from build123d import *

# Parameters (mm, degrees)
F1_DEPTH = 63.5
F2_DEPTH = 25.4
F3_DEPTH = 10.4775
F0_W     = 25.4
F0_H     = 4.7752
F0_H_2   = 19.05
F0_H_3   = 4.7498
F5_R     = 5.08


with BuildPart() as f1:
    # F0 (on Front) → F1 (new body, symmetric)
    with BuildSketch(Plane.XZ):
        Polygon((22.225, 9.525), (-41.275, 9.525), (-41.275, -9.525), (41.275, -9.525), (41.275, 9.525), align=None)
    extrude(amount=F1_DEPTH, both=True)

    # F0 (on Front) → F2 (join, symmetric)
    with BuildSketch(Plane.XZ):
        Polygon((22.225, 9.525), (-41.275, 9.525), (-41.275, -9.525), (41.275, -9.525), (41.275, 9.525), align=None)
        with BuildLine():
            Line((22.225, 27.0002), (22.225, 9.525))
            Line((22.225, 9.525), (41.275, 9.525))
            Line((41.275, 9.525), (41.275, 27.0002))
            ThreePointArc((41.275, 27.0002), (45.9246798487, 38.2255201513), (57.15, 42.8752))
            Line((57.15, 42.8752), (85.725, 42.8752))
            Line((85.725, 42.8752), (85.725, 61.9252))
            Line((85.725, 61.9252), (57.15, 61.9252))
            ThreePointArc((57.15, 61.9252), (32.4542956671, 51.6959043329), (22.225, 27.0002))
        make_face()
    extrude(amount=F2_DEPTH, both=True)

    # F0 (on Front) → F3 (join, symmetric)
    with BuildSketch(Plane.XZ):
        with BuildLine():
            add(Edge.make_bspline(
                [(-41.275, 9.525), (-41.4362549782, 59.2387728393), (7.6155788265, 61.9246140122), (57.15, 61.9252)],
                knots=[0, 0, 0, 0, 111.5045361635, 111.5045361635, 111.5045361635, 111.5045361635], degree=3))
            Line((-41.275, 9.525), (22.225, 9.525))
            Line((22.225, 9.525), (22.225, 27.0002))
            ThreePointArc((22.225, 27.0002), (32.4542956671, 51.6959043329), (57.15, 61.9252))
        make_face()
    extrude(amount=F3_DEPTH, both=True)

    # F0 (on Front) → F4 (revolve)
    with BuildSketch(Plane.XZ):
        with Locations((98.425, 40.4876)):
            Rectangle(F0_W, F0_H)
        with Locations((98.425, 52.4002)):
            Rectangle(F0_W, F0_H_2)
        with Locations((98.425, 64.3001)):
            Rectangle(F0_W, F0_H_3)
    revolve(axis=Axis((85.725, 0, 52.3875), (0, 0, 1)))

    # F5
    f5_edges = [f1.edges().sort_by_distance(p)[0] for p in [
        (41.275, 63.5, 0),
        (-41.275, 63.5, 0),
        (-41.275, -63.5, 0),
        (41.275, -63.5, 0),
    ]]
    fillet(f5_edges, radius=F5_R)


solid = f1.part
Model file for the job. Use its own axes, mm. A direction names the side the tool comes from. Coordinates: 2 decimals unless noted, no trailing zeros. Write each loop counter-clockwise with the first axis right and the second up, starting at its lowest first coordinate (ties: lowest second). Pieces come first, ordered by that corner, then holes. Notation, with made-up numbers: (-14, 23) - (6, 23) arc R9 ccw to (6, 40) - close; hole circle Ø8 at (15.25, 2.25). An arc over 180 degrees is marked (long way). Write each question's results on one line, items separated by ' | '. Start each with the question number.
1) Cut at A-A (y = 13). Write the cut outline in (x, z) (3 decimals).
2) Probe line 1 along Z through (x, y) = (-11.5, 19) (3 decimals); line 2 along Y through (x, z) = (-15, 50.5); line 3 along X through (y, z) = (0, 12) (3 decimals). List the from-to ranges inside material, lowest first. Write a range as from..to.
3) Flat gauge pins, fed straight in: P1, Ø7.5, axis at y = 18.5, z = 15.5, coming from the -X side (3 decimals); P2, Ø5, axis at x = -9.5, y = 2, coming from the +Z side; P3, Ø5, axis at x = 13.5, y = 15.5, coming from the +Z side (3 decimals); P4, Ø15.5, axis at x = 69, z = 24, coming from the -Y side. Where does each tip first touch, or does it go through?
4) 3-axis set-ups, long thin cutter, end or side, ignore diameter. For faces 1 (the face through (22.225, 18, 18)), 2 (the face through (46, 25.4, 42)), 3 (the face through (22.225, -18, 18)), 4 (the face through (41.275, -1, 4)), 5 (the face through (60, -2, 61.925)): which of +Z, -Z, +X, -X, +Y, -Y reach the whole face in a straight line?
5) Cut at D-D (x = 101). Write the cut outline in (y, z) (3 decimals).
6) Cut at C-C (y = 39.5). Write the cut outline in (x, z) (3 decimals), then the cut area to 3 significant figures.
7) Cut at B-B (z = -2). Write the cut outline in (x, y) (3 decimals).
Returned:
1) outline: (-41.275, -9.525) - (41.275, -9.525) - (41.275, 27) arc R15.875 cw to (57.15, 42.875) - (63.904, 42.875) - (63.904, 38.1) - (107.546, 38.1) - (107.546, 66.675) - (63.904, 66.675) - (63.904, 61.925) - (57.15, 61.925) arc R34.925 ccw to (22.225, 27) - (22.225, 9.525) - (-41.275, 9.525) - close
2) line 1: -9.525..9.525 | line 2: -10.48..10.48 | line 3: -41.241..41.275
3) P1: x = 22.225 | P2: z = 55.64 | P3: z = 9.525 | P4: through
4) face 1: +Z, -X, +Y | face 2: +Z, +X, -X, +Y | face 3: +Z, -X, -Y | face 4: -Z, +X, +Y, -Y | face 5: +Z, -X
5) outline: (-20.294, 38.1) - (20.294, 38.1) - (20.294, 66.675) - (-20.294, 66.675) - close
6) outline: (-41.275, -9.525) - (41.275, -9.525) - (41.275, 9.525) - (-41.275, 9.525) - close | area: 1,570 mm^2
7) outline: (-41.275, -58.42) arc R5.08 ccw to (-36.195, -63.5) - (36.195, -63.5) arc R5.08 ccw to (41.275, -58.42) - (41.275, 58.42) arc R5.08 ccw to (36.195, 63.5) - (-36.195, 63.5) arc R5.08 ccw to (-41.275, 58.42) - close
